Check sheet for the modelled part. Datum: model origin and axes. Units: mm. A direction names the side the tool comes from. Coordinates: 2 decimals unless noted, no trailing zeros. Order: outer loops, then holes, each group sorted by start corner. A loop starts at its lowest first (then second) coordinate and runs counter-clockwise, first axis right, second up.
1. Cross-section at C-C (z = 0). Enter the section's corners in (x, y).
2. Cross-section at B-B (y = -5.35). Enter the section's corners in (x, z), then the cut area to 3 significant figures.
3. Thickness scan on line 1 (Z direction, x = 19, y = -0.45); line 2 (X direction, y = -3.65, z = 0); line 3 (X direction, y = -1.8, z = -2.5). Record the ranges inside material, lowest first.
4. Set-up check for faces 4 (the cylindrical face through (-30, -3, 0)), 5 (the flat face through (0, -3, -6.5)): record each of +Z, -Z, +X, -X, +Y, -Y from which the full face is reachable in a straight line by a thin tool's end or side.
5. Cross-section at A-A (x = -10.5). Enter the section's corners in (y, z), then the cut area to 3 significant figures.
6. Gauge pin test, flat end, axial feed: pin 1 Ø1.5 at (x, z) = (14.5, -4) entering from +Y. Record the tip position at first contact, or that the pin passes through.
7. Draft check along Z on faces 1 (the cylindrical face through (-30.5, -3, 0.1)), 2 (the flat face through (0, -3, -6)), 3 (the flat face through (-0.1, 0, -6.2)). Enter one of: released by +Z, released by -Z, zero draft, split by the parting line, or undercut.
```python
from build123d import *

# Parameters (mm, degrees)
F1_DEPTH = 6


with BuildPart() as f1:
    # F0 (on Front) → F1 (new body)
    with BuildSketch(Plane.XZ):
        with BuildLine():
            Line((0, 6.5), (-24, 6.5))
            ThreePointArc((-24, 6.5), (-30.5, 0), (-24, -6.5))
            Line((-24, -6.5), (0, -6.5))
            Line((0, -6.5), (24, -6.5))
            ThreePointArc((24, -6.5), (30.5, 0), (24, 6.5))
            Line((24, 6.5), (0, 6.5))
        make_face()
        with BuildLine():
            ThreePointArc((-24, -6), (-30, 0), (-24, 6))
            Line((-24, 6), (0, 6))
            Line((0, 6), (24, 6))
            ThreePointArc((24, 6), (30, 0), (24, -6))
            Line((24, -6), (0, -6))
            Line((0, -6), (-24, -6))
        make_face(mode=Mode.SUBTRACT)
    extrude(amount=F1_DEPTH)


solid = f1.part
```
Data:
1. outline: (-30.5, -6) - (-30, -6) - (-30, 0) - (-30.5, 0) - close; (30, -6) - (30.5, -6) - (30.5, 0) - (30, 0) - close
2. outline: (-24, -6.5) - (24, -6.5) arc R6.5 ccw to (24, 6.5) - (-24, 6.5) arc R6.5 ccw to start; hole (-24, -6) - (24, -6) arc R6 ccw to (24, 6) - (-24, 6) arc R6 ccw to start
2. area: 67.6 mm2
3. line 1: z = -6.5 to -6, 6 to 6.5
3. line 2: x = -30.5 to -30, 30 to 30.5
3. line 3: x = -30 to -29.45, 29.45 to 30
4. face 4: +Y, -Y
4. face 5: -Z, +X, -X, +Y, -Y
5. outline: (-6, -6.5) - (0, -6.5) - (0, -6) - (-6, -6) - close; (-6, 6) - (0, 6) - (0, 6.5) - (-6, 6.5) - close
5. area: 6.00 mm2
6. pin 1: passes through
7. face 1: split by the parting line
7. face 2: undercut
7. face 3: zero draft
